Work out the finished part from the listing and answer in its coordinate system (mm). Give positions to 0.01 mm unless a question says otherwise; leave off trailing zeros. Write each loop counter-clockwise with the first axis right and the second up, starting at its lowest first coordinate (ties: lowest second). Pieces come first, ordered by that corner, then holes. Notation, with made-up numbers: (7, 27.25) - (15, 27.25) arc R22 ccw to (15, 58.25) - close; hole circle Ø10 at (0, -12). An arc over 180 degrees is marked (long way). Write item = value, one per line.
from build123d import *

# Parameters (mm, degrees)
BOSS_EXTRU_1_DEPTH      = 44
ENL_V_MAT_EXTRU_1_REACH = 458
ESQUISSE2_R             = 1.75


with BuildPart() as part:
    # Esquisse1 → Boss.-Extru.1 (new body)
    with BuildSketch(Plane.XY):
        Polygon((-44, 1000), (-500, 0), (-451.641297619, 0), (-44, 893.950214076), align=None)
    extrude(amount=BOSS_EXTRU_1_DEPTH)

    # Enlèv. mat.-Extru.1: up to this face of the body (flat: up to its plane)
    enl_v_mat_extru_1_end = Plane(part.part.faces().sort_by_distance((-272, 500, 22))[0])
    # Esquisse2 → Enlèv. mat.-Extru.1 (cut, up to the picked face)
    with BuildSketch(Plane(origin=(-44, 0, 0), x_dir=(0, 0, -1), z_dir=(1, 0, 0)), mode=Mode.PRIVATE) as enl_v_mat_extru_1_sk1:
        with Locations((-22, 950)):
            Circle(ESQUISSE2_R)
    enl_v_mat_extru_1_tool1 = split(extrude(enl_v_mat_extru_1_sk1.sketch, amount=-ENL_V_MAT_EXTRU_1_REACH, mode=Mode.PRIVATE), bisect_by=enl_v_mat_extru_1_end, keep=Keep.BOTH, mode=Mode.PRIVATE)
    add(enl_v_mat_extru_1_tool1.solids().sort_by_distance((-44, 950, 22))[0], mode=Mode.SUBTRACT)


solid = part.part
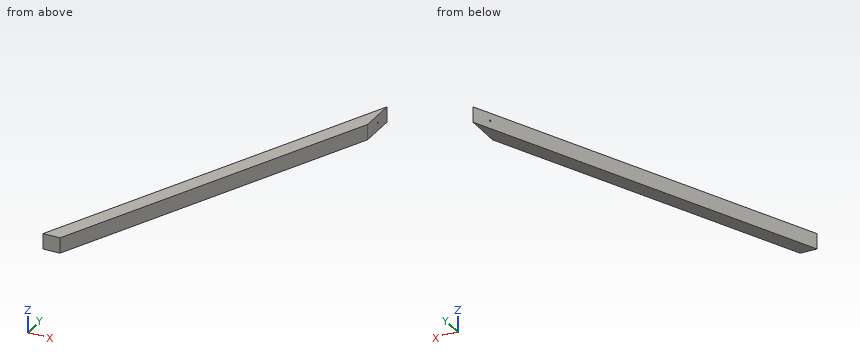
1. Find section A-A, the plane x = -122. Give the vertices of the cut face in (y, z).
Solution:
outline = (722.9, 0) - (828.95, 0) - (828.95, 44) - (722.9, 44) - close
2. Find section B-B, the plane y = 644. Give the vertices of the cut face in (x, z).
Solution:
outline = (-206.34, 0) - (-157.98, 0) - (-157.98, 44) - (-206.34, 44) - close
3. Given pin 1 (8 mm diameter, centred on x = -271.5, z = 35, fed in from -Y); pin 2 (3 mm diameter, centred on x = -224.5, z = 26.5, fed in from -Y); pin 3 (5 mm diameter, centred on y = 541.5, z = 34, fed in from +X), each flat-ended and moving along its own axis, determine where each tip first touches the part or whether it passes through.
Solution:
pin_1 = 386.27
pin_2 = 494.83
pin_3 = -203.58
4. Straight lines are drawn through the part: line 1 (Z direction, x = -57, y = 950); line 2 (Y direction, x = -49.5, z = 22); line 3 (Y direction, x = -438, z = 7). For each, find the intervals that lie inside material, in ascending order.
Solution:
line_1 = 0 to 20.25, 23.75 to 44
line_2 = 881.89 to 948.25, 951.75 to 987.94
line_3 = 29.92 to 135.96
